Geometry check sheet. Reference: the model listing, model coordinates, mm. Round coordinates to 2 decimals unless told otherwise and drop trailing zeros. Order: outer loops, then holes, each group sorted by start corner. A loop starts at its lowest first (then second) coordinate and runs counter-clockwise, first axis right, second up. Notation, with made-up numbers: (89, 51) - (132, 51) arc R26 ccw to (132, 87) - close; hole circle Ø3 at (-28, 27.25). An arc over 180 degrees is marked (long way). Write each question's results on one line, items separated by ' | '.
```python
from build123d import *

# Parameters (mm, degrees)
SKETCH1_R                           = 152.4
SKETCH1_R_2                         = 63.5
THRUSTPLATE_TC3_DEPTH               = 12.7
UNDEF_CLEARANCE_THRUSTPLATE_D       = 13.89126
CLEARANCE_THRUSTPLATE_PATTERN_COUNT = 4
F_10_CLEARANCE_HOLE1_D              = 5.1054
CIRPATTERN1_COUNT                   = 10
CUT_EXTRUDE1_REACH                  = 217.9


with BuildPart() as part:
    # Sketch1 → ThrustPlate_TC3 (new body)
    with BuildSketch(Plane(origin=(0, 0, 0), x_dir=(1, 0, 0), z_dir=(0, 1, 0))):
        with Locations(Location((0, 0, 0), (0, 0, 270))):
            Circle(SKETCH1_R)
        with Locations(Location((0, 0, 0), (0, 0, 270))):
            Circle(SKETCH1_R_2, mode=Mode.SUBTRACT)
    extrude(amount=-THRUSTPLATE_TC3_DEPTH)

    # UNDEF_Clearance_ThrustPlate (through all)
    with Locations(Plane(origin=(0, 0, 0), x_dir=(1, 0, 0), z_dir=(0, 1, 0))):
        with Locations((0, 127)):
            undef_clearance_thrustplate = Hole(UNDEF_CLEARANCE_THRUSTPLATE_D / 2)

    # Clearance_ThrustPlate_Pattern: UNDEF_Clearance_ThrustPlate ×4 about axis
    clearance_thrustplate_pattern_axis = Axis((0, 0, 0), (0, 1, 0))
    for i in range(1, CLEARANCE_THRUSTPLATE_PATTERN_COUNT):
        add(undef_clearance_thrustplate.rotate(clearance_thrustplate_pattern_axis, i * 360 / CLEARANCE_THRUSTPLATE_PATTERN_COUNT), mode=Mode.SUBTRACT)

    # #10 Clearance Hole1 (through all)
    with Locations(Plane(origin=(0, 0, 0), x_dir=(1, 0, 0), z_dir=(0, 1, 0))):
        with Locations((0, 73.025)):
            f_10_clearance_hole1 = Hole(F_10_CLEARANCE_HOLE1_D / 2)

    # CirPattern1: #10 Clearance Hole1 ×10 about axis
    cirpattern1_axis = Axis((0, 0, 0), (0, 1, 0))
    for i in range(1, CIRPATTERN1_COUNT):
        add(f_10_clearance_hole1.rotate(cirpattern1_axis, i * 360 / CIRPATTERN1_COUNT), mode=Mode.SUBTRACT)

    # Sketch24 → Cut-Extrude1 (cut, up to next)
    with BuildSketch(Plane(origin=(0, 0, 0), x_dir=(1, 0, 0), z_dir=(0, 1, 0)), mode=Mode.PRIVATE) as cut_extrude1_sk1:
        with BuildLine():
            ThreePointArc((-45.123199962, 48.17827493), (-64.72944972, 47.028698036), (-59.764097944, 28.026807647))
            ThreePointArc((-59.764097944, 28.026807647), (-58.45757522, 26.637277771), (-58.48647188, 24.73019626))
            ThreePointArc((-58.48647188, 24.73019626), (-51.372579143, 37.324363521), (-41.593128054, 47.981889278))
            ThreePointArc((-41.593128054, 47.981889278), (-43.397940793, 47.365086324), (-45.123199962, 48.17827493))
        make_face()
    cut_extrude1_tool1 = extrude(cut_extrude1_sk1.sketch, amount=-CUT_EXTRUDE1_REACH, mode=Mode.PRIVATE) & part.part
    add(cut_extrude1_tool1.solids().sort_by_distance((-57.000167, 0, -41.413046))[0], mode=Mode.SUBTRACT)


solid = part.part
```
(1) Draft check along Z on faces 1 (the face through (2, 0, 66)), 2 (the face through (-92.73, -6.26, -120.94)), 3 (the face through (-64.54, -6.26, -47.28)). Enter one of: released by +Z, released by -Z, zero draft, split by the parting line, or undercut.
Answers follow:
face 1: zero draft | face 2: split by the parting line | face 3: undercut
(2) Material ranges on line 1 (X direction, y = -8.75, z = 0); line 2 (X direction, y = -12, z = 24); line 3 (Z direction, x = 8.5, y = -6.5), recorded low to high.
Answers follow:
line 1: -152.4 to -133.95, -120.05 to -63.5, 63.5 to 120.05, 133.95 to 152.4 | line 2: -150.5 to -71.56, -67.34 to -58.79, 58.79 to 67.34, 71.56 to 150.5 | line 3: -152.16 to -62.93, 62.93 to 152.16
(3) Section check B-B (z = 0). Record the cut outline in (x, y), then the cut area to 3 significant figures.
Answers follow:
outline: (-152.4, -12.7) - (-133.95, -12.7) - (-133.95, 0) - (-152.4, 0) - close; (-120.05, -12.7) - (-63.5, -12.7) - (-63.5, 0) - (-120.05, 0) - close; (63.5, -12.7) - (120.05, -12.7) - (120.05, 0) - (63.5, 0) - close; (133.95, -12.7) - (152.4, -12.7) - (152.4, 0) - (133.95, 0) - close | area: 1,910 mm²
(4) Section check D-D (y = -9.75). Give the number of separate pieces and of enclosed holes in the cut face, then the cut area to 3 significant figures.
Answers follow:
separate pieces: 1 | enclosed holes: 15 | area: 59,100 mm²
(5) Depth check by flat-ended pin: pin 1 Ø3 at (y, z) = (-9, 51) entering from -X; pin 2 Ø4 at (x, y) = (-118, -5) entering from -Z. Enter the tip coordinate at first touch or a pass-through.
Answers follow:
pin 1: x = -144.14 | pin 2: z = -98.84
(6) Section check A-A (x = 13). Record the cut outline in (y, z).
Answers follow:
outline: (-12.7, -151.84) - (0, -151.84) - (0, -62.16) - (-12.7, -62.16) - close; (-12.7, 62.16) - (0, 62.16) - (0, 151.84) - (-12.7, 151.84) - close
(7) Section check C-C (z = 32.5). Record the cut outline in (x, y).
Answers follow:
outline: (-148.89, -12.7) - (-54.55, -12.7) - (-54.55, 0) - (-148.89, 0) - close; (54.55, -12.7) - (148.89, -12.7) - (148.89, 0) - (54.55, 0) - close
